Here's how the part is built. I have some questions about the finished solid (model axes, mm). Face numbers are marked on the shaded views. A direction names the side the tool comes from. Coordinates: 2 decimals unless noted, no trailing zeros. Write each loop counter-clockwise with the first axis right and the second up, starting at its lowest first coordinate (ties: lowest second). Pieces come first, ordered by that corner, then holes.
```python
from build123d import *

# Parameters (mm, degrees)
SKETCH1_W                 = 14.7
SKETCH1_H                 = 14.7
BOSS_EXTRUDE1_DEPTH       = 76.2
SKETCH6_R                 = 3.175
CUT_EXTRUDE4_DEPTH        = 78.952244997
CHAMFER5_SIZE             = 1
CHAMFER6_SIZE             = 2.54
BOSS_EXTRUDE2_DEPTH       = 15
BOSS_EXTRUDE2_DEPTH_BACK  = 29.7
SKETCH4_W                 = 35.56
SKETCH4_H                 = 20.32
SKETCH5_R                 = 3.175
TRAYSUPPORTMOUNTING_DEPTH = 106.262274819
CHAMFER4_SIZE             = 1
CUT_EXTRUDE2_REACH        = 102.657
SKETCH3_R                 = 3.175
FILLET1_R                 = 6.35


with BuildPart() as part:
    # Sketch1 → Boss-Extrude1 (new body)
    with BuildSketch(Plane(origin=(0, 0, 0), x_dir=(1, 0, 0), z_dir=(0, 1, 0))):
        Rectangle(SKETCH1_W, SKETCH1_H)
    extrude(amount=BOSS_EXTRUDE1_DEPTH)

    # Sketch6 → Cut-Extrude4 (cut, through all)
    with BuildSketch(Plane(origin=(7.35, 0, 0), x_dir=(0, 0, -1), z_dir=(1, 0, 0))):
        with Locations((0, 65.405)):
            Circle(SKETCH6_R)
        with Locations((0, 51.435)):
            Circle(SKETCH6_R)
        with Locations((0, 37.465)):
            Circle(SKETCH6_R)
        with Locations((0, 23.495)):
            Circle(SKETCH6_R)
        with Locations((0, 9.525)):
            Circle(SKETCH6_R)
    extrude(amount=-CUT_EXTRUDE4_DEPTH, mode=Mode.SUBTRACT)

    # Chamfer5
    chamfer5_edges = [part.edges().sort_by_distance(p)[0] for p in [
        (-7.35, 65.405, 3.175),
        (7.35, 65.405, 3.175),
        (-7.35, 51.435, 3.175),
        (7.35, 51.435, 3.175),
        (-7.35, 37.465, 3.175),
        (7.35, 37.465, 3.175),
        (-7.35, 23.495, 3.175),
        (7.35, 23.495, 3.175),
    ]]
    chamfer(chamfer5_edges, length=CHAMFER5_SIZE)

    # Chamfer6
    chamfer6_edges = [part.edges().sort_by_distance(p)[0] for p in [
        (0, 0, -7.35),
        (7.35, 0, 0),
        (0, 0, 7.35),
        (-7.35, 0, 0),
    ]]
    chamfer(chamfer6_edges, length=CHAMFER6_SIZE)

    # Sketch4 → Boss-Extrude2 (add, two sides: drawn at the far end of the back side and taken through both)
    with BuildSketch(Plane.XY.offset(7.35).offset(-BOSS_EXTRUDE2_DEPTH_BACK)):
        with Locations((0, 86.36)):
            Rectangle(SKETCH4_W, SKETCH4_H)
    extrude(amount=BOSS_EXTRUDE2_DEPTH + BOSS_EXTRUDE2_DEPTH_BACK)

    # Sketch5 → TraySupportMounting (cut, through all)
    with BuildSketch(Plane(origin=(17.78, 0, 0), x_dir=(0, 0, -1), z_dir=(1, 0, 0))):
        with Locations((16, 88.9)):
            Circle(SKETCH5_R)
        with Locations((4.57, 88.9)):
            Circle(SKETCH5_R)
    extrude(amount=-TRAYSUPPORTMOUNTING_DEPTH, mode=Mode.SUBTRACT)

    # Chamfer4
    chamfer4_edges = [part.edges().sort_by_distance(p)[0] for p in [
        (-17.78, 88.9, -12.825),
        (17.78, 88.9, -12.825),
        (-17.78, 88.9, -1.395),
        (17.78, 88.9, -1.395),
    ]]
    chamfer(chamfer4_edges, length=CHAMFER4_SIZE)

    # Sketch3 → Cut-Extrude2 (cut, up to next)
    with BuildSketch(Plane(origin=(0, 96.52, 0), x_dir=(1, 0, 0), z_dir=(0, 1, 0)), mode=Mode.PRIVATE) as cut_extrude2_sk1:
        with Locations(Location((0, -14.095, 0), (0, 0, 270))):
            Circle(SKETCH3_R)
    cut_extrude2_tool1 = extrude(cut_extrude2_sk1.sketch, amount=-CUT_EXTRUDE2_REACH, mode=Mode.PRIVATE) & part.part
    add(cut_extrude2_tool1.solids().sort_by_distance((0, 96.52, 14.095))[0], mode=Mode.SUBTRACT)

    # Fillet1
    fillet1_edges = [part.edges().sort_by_distance(p)[0] for p in [
        (-17.78, 86.36, 22.35),
        (17.78, 86.36, 22.35),
    ]]
    fillet(fillet1_edges, radius=FILLET1_R)


solid = part.part
```
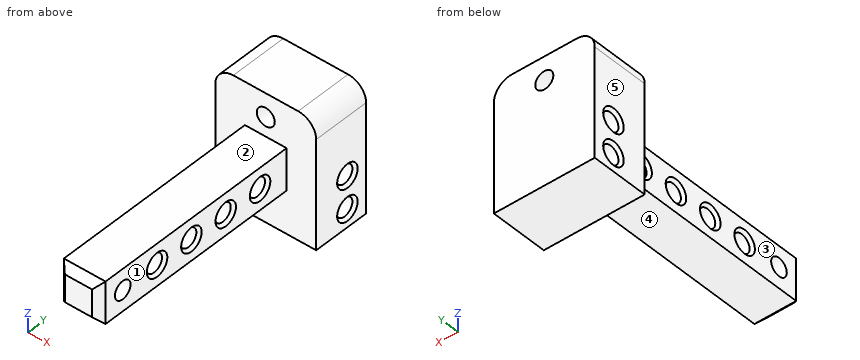
1) Will these pins go through, and if not, where does the flat tip stop? pin 1 (16 mm diameter, centred on y = 26.5, z = -1.5, fed in from -X); pin 2 (16 mm diameter, centred on x = -3.5, y = 42.5, fed in from +Z); pin 3 (7.5 mm diameter, centred on y = 23.495, z = 0, fed in from +X) (3 decimals).
Values follow:
pin 1: stops at x = -7.35
pin 2: stops at z = 7.35
pin 3: stops at x = 6.925
2) Imagine slicing it at C-C on x = 0. Count the separate pieces of the cut face and the enclosed holes in it, then the cut area to 3 significant figures.
Values follow:
separate pieces: 2
enclosed holes: 7
area: 1,670 mm2
3) I need wall thicknesses on probe 1 along Y at (x, z) = (0, 0); probe 2 along Z at (x, y) = (9.5, 88); probe 3 along Y at (x, z) = (-15, 19.5). Which ranges of each line are inside material? Lowest first, please.
Values follow:
probe 1: y = 0 to 6.35, 12.7 to 20.32, 26.67 to 34.29, 40.64 to 48.26, 54.61 to 62.23, 68.58 to 96.52
probe 2: z = -22.35 to -19.04, -12.96 to -7.61, -1.53 to 22.35
probe 3: y = 76.2 to 96.52
4) Imagine slicing it at A-A on y = 88.9. Please give me the cut outline in (x, z) (3 decimals), then the cut area to 3 significant figures.
Values follow:
outline: (-17.78, -22.35) - (17.78, -22.35) - (17.78, -20.175) - (16.78, -19.175) - (-16.78, -19.175) - (-17.78, -20.175) - close; (-17.78, -11.825) - (-16.78, -12.825) - (16.78, -12.825) - (17.78, -11.825) - (17.78, -8.745) - (16.78, -7.745) - (-16.78, -7.745) - (-17.78, -8.745) - close; (-17.78, -0.395) - (-16.78, -1.395) - (16.78, -1.395) - (17.78, -0.395) - (17.78, 16) arc R6.35 ccw to (11.43, 22.35) - (-11.43, 22.35) arc R6.35 ccw to (-17.78, 16) - close; hole circle Ø6.35 at (0, 14.095)
area: 1,080 mm2
5) Imagine slicing it at D-D on x = -12.5. Please give me the cut outline in (y, z) (3 decimals).
Values follow:
outline: (76.2, -22.35) - (96.52, -22.35) - (96.52, 22.259) - (76.2, 22.259) - close; hole circle Ø6.35 at (88.9, -16); hole circle Ø6.35 at (88.9, -4.57)
6) Imagine slicing it at B-B on z = -16. Please give me the cut outline in (x, y) (3 decimals).
Values follow:
outline: (-17.78, 76.2) - (17.78, 76.2) - (17.78, 84.725) - (16.78, 85.725) - (-16.78, 85.725) - (-17.78, 84.725) - close; (-17.78, 93.075) - (-16.78, 92.075) - (16.78, 92.075) - (17.78, 93.075) - (17.78, 96.52) - (-17.78, 96.52) - close
7) On a 3-axis mill with a long thin cutter (end or side, diameter ignored), from which of +Z, -Z, +X, -X, +Y, -Y can I reach the whole of each face in a straight line? I mean the marked faces 1, 2, 3, 4 and 5. Say none if no direction works.
Values follow:
face 1: +Z, -Z, +X, -Y
face 2: +Z, +X, -X, -Y
face 3: +Z, -Z, -X, -Y
face 4: -Z, +X, -X, -Y
face 5: +Z, -Z, -X, +Y, -Y
